```python
from build123d import *

# Parameters (mm, degrees)
ESQUISSE1_R                  = 7.499999999999999
BOSS_EXTRU_1_DEPTH           = 50
COQUE1_T                     = -3
ESQUISSE2_R                  = 3.25
ENL_V_MAT_EXTRU_1_DEPTH      = 3
ENL_V_START                  = 3.741658222
ENL_V_MAT_EXTRU_2_DEPTH      = 3.758341878
ENL_V_MAT_EXTRU_3_DEPTH      = 52.1126209805562
ENL_V_MAT_EXTRU_3_DEPTH_BACK = 52.1126209805562
ESQUISSE5_RX                 = 6.5
ESQUISSE5_RY                 = 5.25


# Read off the part's stored shape, not the designer's step: Enlèv. mat.-Extru.2
with BuildPart() as part:
    # Esquisse1 → Boss.-Extru.1 (new body)
    with BuildSketch(Plane.XY):
        Circle(ESQUISSE1_R)
    extrude(amount=BOSS_EXTRU_1_DEPTH)

    # Coque1
    coque1_openings = [part.faces().sort_by_distance(p)[0] for p in [
        (0, 0, 50),
    ]]
    offset(amount=COQUE1_T, openings=coque1_openings, kind=Kind.INTERSECTION)

    # Esquisse2 → Enlèv. mat.-Extru.1 (cut)
    with BuildSketch(Plane(origin=(0, 0, 0), x_dir=(-1, 0, 0), z_dir=(0, 0, -1))):
        Circle(ESQUISSE2_R)
    extrude(amount=-ENL_V_MAT_EXTRU_1_DEPTH, mode=Mode.SUBTRACT)

    # Enlèv. mat.-Extru.2 outline → Enlèv. mat.-Extru.2 (cut)
    with BuildSketch(Plane(origin=(0, 0, 0), x_dir=(1, 0, 0), z_dir=(0, 1, 0)).offset(ENL_V_START)):
        with BuildLine():
            add(Edge.make_bspline(
                [(0, -4.5), (-0.665777373921639, -4.5), (-1.3108797918298, -4.77502806566904), (-2.22588234313574, -5.69066668426073), (-2.49954115482472, -6.34073255596721), (-2.50045763095517, -7.65578287810988), (-2.2278471774147, -8.30775806725704), (-1.30741263251952, -9.22804991342628), (-0.656855076796676, -9.49973692434233), (0.654851008774013, -9.5002626740288), (1.30573460063621, -9.2296895812874), (2.22937932360176, -8.306264256457), (2.49994577794749, -7.65925317637901), (2.50005420513552, -6.34115812623399), (2.22645885760644, -5.69117807090988), (1.31005066740923, -4.77426391153354), (0.665777373921637, -4.5), (0, -4.5)],
                knots=[0, 0, 0, 0, 0.125, 0.125, 0.25, 0.25, 0.375, 0.375, 0.5, 0.5, 0.625, 0.625, 0.75, 0.75, 0.875, 0.875, 1, 1, 1, 1], degree=3))
        make_face()
    extrude(amount=ENL_V_MAT_EXTRU_2_DEPTH, mode=Mode.SUBTRACT)

    # Esquisse5 → Enlèv. mat.-Extru.3 (cut, two sides: drawn at the far end of the back side and taken through both)
    with BuildSketch(Plane(origin=(0, 0, 0), x_dir=(1, 0, 0), z_dir=(0, 1, 0)).offset(-ENL_V_MAT_EXTRU_3_DEPTH_BACK)):
        with Locations(Location((0, -50), (0, 0, -90))):
            Ellipse(ESQUISSE5_RX, ESQUISSE5_RY)
    extrude(amount=ENL_V_MAT_EXTRU_3_DEPTH + ENL_V_MAT_EXTRU_3_DEPTH_BACK, mode=Mode.SUBTRACT)


solid = part.part
```
Input: part model. Units: mm. Frame: model coordinates. A direction names the side the tool comes from. Coordinates: 2 decimals unless noted, no trailing zeros. Loops run counter-clockwise (first coordinate to the right, second up) from the corner with the lowest first, then second, coordinate; pieces in that order, holes last. Notation, with made-up numbers: M -26.75,-38.5 L 18.25,-38.5 A14 cw 18.25,-19.5 Z; hole C 79.5,-14 d5. An arc over 180 degrees is marked long. One line per item, written item: value.
(1) Pin query (flat end, axial travel): pin 1 (6 mm diameter, centred on y = 4.5, z = 41.5, fed in from -X); pin 2 (1 mm diameter, centred on x = 2.5, z = 22, fed in from +Y); pin 3 (1.5 mm diameter, centred on y = -4.5, z = 30, fed in from +X); pin 4 (5.5 mm diameter, centred on x = 0, y = 0, fed in from +Z). Return the tip coordinate at first contact, or that it passes through.
Filled in:
pin 1: x = -7.35
pin 2: y = 7.23
pin 3: x = 6.5
pin 4: through
(2) Reachability of faces 4 (the flat face through (-6, 0, 50)), 5 (the cylindrical face through (2.08, -3.99, 24.52)) from +Z, -Z, +X, -X, +Y, -Y: full face, straight path, thin tool, end or side. Return the list, or none.
Filled in:
face 4: +Z, +X, -X, +Y, -Y
face 5: +Z
(3) Section B-B (x = 0.5). Give the number of separate pieces and of enclosed holes in the cut face, and give its area (3 significant figures).
Filled in:
separate pieces: 3
enclosed holes: 0
area: 255 mm^2
(4) Line query: line 1 along Y through (x, z) = (0, 29.5); line 2 along Y through (x, z) = (0, 1.15); line 3 along X through (y, z) = (-6, 41.5). Output: solid intervals per line, ascending. Write a range as from..to.
Filled in:
line 1: -7.5..-4.5, 4.5..7.5
line 2: -7.5..-3.25, 3.25..7.5
line 3: -4.5..4.5
(5) Pull-direction query (Y, two-part tool) for faces 1 (the flat face through (6, 0, 50)), 2 (the cylindrical face through (2.579, -1.978, 1.479)), 3 (the cylindrical face through (-1.63, -7.32, 24.65)); classes: +Y half, -Y half, draft (parallel to the pull), parting line (faces both ways), or undercut.
Filled in:
face 1: draft
face 2: undercut
face 3: parting line
(6) Section A-A (z = 10.5). Output: boundary loops of the cut face in (x, y), and give its area (3 significant figures).
Filled in:
outline: C 0,0 d15; hole C 0,0 d9
area: 113 mm^2
